Source: CAD feature listing. Evaluate the final solid. Frame: model axes, mm. A direction names the side the tool comes from. Give positions to 0.01 mm unless a question says otherwise; leave off trailing zeros. Order: outer loops, then holes, each group sorted by start corner. A loop starts at its lowest first (then second) coordinate and runs counter-clockwise, first axis right, second up. Notation, with made-up numbers: (-33.5, 78.25) - (8.5, 78.25) arc R25 ccw to (8.5, 96.25) - close; hole circle Ø11 at (-35.5, -7). An arc over 180 degrees is marked (long way). Answer as CSV lines item,"result".
```python
from build123d import *

# Parameters (mm, degrees)
SKETCH2_W           = 42.1
SKETCH2_H           = 90
SKETCH2_R           = 11.75
BOSS_EXTRUDE1_DEPTH = 3
SKETCH3_W           = 42.1
SKETCH3_H           = 90
SKETCH3_R           = 3.5
BOSS_EXTRUDE2_DEPTH = 5
SKETCH6_R           = 0.8
CUT_EXTRUDE1_DEPTH  = 9
SKETCH7_R           = 2.5
CUT_EXTRUDE2_DEPTH  = 9


with BuildPart() as part:
    # Sketch2 → Boss-Extrude1 (new body)
    with BuildSketch(Plane.XY):
        with Locations((0, 23.95)):
            Rectangle(SKETCH2_W, SKETCH2_H)
        Circle(SKETCH2_R, mode=Mode.SUBTRACT)
    extrude(amount=BOSS_EXTRUDE1_DEPTH)

    # Sketch3 → Boss-Extrude2 (add)
    with BuildSketch(Plane.XY.offset(3)):
        with Locations((0, 23.95)):
            Rectangle(SKETCH3_W, SKETCH3_H)
        Circle(SKETCH3_R, mode=Mode.SUBTRACT)
    extrude(amount=BOSS_EXTRUDE2_DEPTH)

    # Sketch6 → Cut-Extrude1 (cut, through all)
    with BuildSketch(Plane.XY.offset(8)):
        with Locations((-15.5, 15.5)):
            Circle(SKETCH6_R)
        with Locations((-15.5, -15.5)):
            Circle(SKETCH6_R)
        with Locations((15.5, 15.5)):
            Circle(SKETCH6_R)
        with Locations((15.5, -15.5)):
            Circle(SKETCH6_R)
    extrude(amount=-CUT_EXTRUDE1_DEPTH, mode=Mode.SUBTRACT)

    # Sketch7 → Cut-Extrude2 (cut, through all)
    with BuildSketch(Plane.XY.offset(8)):
        with Locations((0, 46.707876994)):
            Circle(SKETCH7_R)
    extrude(amount=-CUT_EXTRUDE2_DEPTH, mode=Mode.SUBTRACT)


solid = part.part
```
(1) Contact query for a flat-ended pin moving along its axis: pin 1 (1 mm diameter, centred on x = 15.5, y = 15.5, fed in from +Z). Output: stop coordinate, or through.
Completed:
pin 1,"through"
(2) Cut plane D-D (z = 6.5). Return loops of the section in (x, y), then the cut area to 3 significant figures.
Completed:
outline,"(-21.05, -21.05) - (21.05, -21.05) - (21.05, 68.95) - (-21.05, 68.95) - close; hole circle Ø1.6 at (-15.5, -15.5); hole circle Ø1.6 at (-15.5, 15.5); hole circle Ø7 at (0, 0); hole circle Ø5 at (0, 46.71); hole circle Ø1.6 at (15.5, -15.5); hole circle Ø1.6 at (15.5, 15.5)"
area,"3,720 mm²"
(3) Ray query, line 1 (Y direction, x = 15.5, z = 3.25); line 2 (Y direction, x = 0, z = 1.5); line 3 (X direction, y = 49, z = 4.5). Return the intervals inside material, ascending. Write a range as from..to.
Completed:
line 1,"-21.05..-16.3, -14.7..14.7, 16.3..68.95"
line 2,"-21.05..-11.75, 11.75..44.21, 49.21..68.95"
line 3,"-21.05..-1, 1..21.05"
(4) Cut plane B-B (y = 15.5). Return loops of the section in (x, z).
Completed:
outline,"(-21.05, 0) - (-16.3, 0) - (-16.3, 8) - (-21.05, 8) - close; (-14.7, 0) - (14.7, 0) - (14.7, 8) - (-14.7, 8) - close; (16.3, 0) - (21.05, 0) - (21.05, 8) - (16.3, 8) - close"
(5) Mould query, pull axis Y, two halves, no side actions, for faces 3 (the flat face through (0, 25, 8)), 4 (the flat face through (0, -21.05, 4)), 5 (the cylindrical face through (14.87, 15.01, 4.06)). Classes: released by +Y, released by -Y, zero draft, split by the parting line, or undercut.
Completed:
face 3,"zero draft"
face 4,"released by -Y"
face 5,"undercut"
(6) Cut plane A-A (x = 0). Return loops of the section in (y, z), then the cut area to 4 significant figures.
Completed:
outline,"(-21.05, 0) - (-11.75, 0) - (-11.75, 3) - (-3.5, 3) - (-3.5, 8) - (-21.05, 8) - close; (3.5, 3) - (11.75, 3) - (11.75, 0) - (44.21, 0) - (44.21, 8) - (3.5, 8) - close; (49.21, 0) - (68.95, 0) - (68.95, 8) - (49.21, 8) - close"
area,"574.5 mm²"
(7) Cut plane C-C (y = 0). Return loops of the section in (x, z), then the cut area to 3 significant figures.
Completed:
outline,"(-21.05, 0) - (-11.75, 0) - (-11.75, 3) - (-3.5, 3) - (-3.5, 8) - (-21.05, 8) - close; (3.5, 3) - (11.75, 3) - (11.75, 0) - (21.05, 0) - (21.05, 8) - (3.5, 8) - close"
area,"231 mm²"
(8) Access query for faces 1 (the flat face through (21.05, 23, 4)), 2 (the flat face through (2.4, 2.8, 3)). Directions: +Z, -Z, +X, -X, +Y, -Y. A direction counts if a zero-diameter tool reaches every point of the face in a straight line with its end or side. Return the directions, or none.
Completed:
face 1,"+Z, -Z, +X, +Y, -Y"
face 2,"-Z"
